Design review of the part shown in the three views and the two pictorial views. Dimensions are in mm from the part's minimum x, y and z. A direction names the side the tool comes from. Coordinates: 2 decimals unless noted, no trailing zeros. Write each loop counter-clockwise with the first axis right and the second up, starting at its lowest first coordinate (ties: lowest second). Pieces come first, ordered by that corner, then holes. Notation, with made-up numbers: (85.5, 35) - (121.5, 35) arc R23 cw to (121.5, 50) - close; hole circle Ø7 at (-13.5, -7). An arc over 180 degrees is marked (long way). Return JSON: item names as keys, results as strings. Group by question number.
(1) We need section C-C on y = 16. State the section outline as (x, z) points.
(2) We need section D-D on z = 225. State the section outline as (x, y) points, then the cut area to 3 significant figures.
(3) To check wall thickness, follow L1, parallel to X at y = 0.85, z = 125; L2, parallel to Y at x = 156.5, z = 31; L3, parallel to X at y = 2.05, z = 225. State the ranges of each line that lie inside material, in increasing order. Write a range as from..to.
(4) We need section A-A on z = 125. State the section outline as (x, y) points.
(5) We need section B-B on x = 125. State the section outline as (y, z) points, then the cut area to 3 significant figures.
(6) For pin 1 Ø1.5 at (x, z) = (125.5, 103) entering from +Y; pin 2 Ø6 at (x, z) = (123.5, 229.5) entering from -Y; pin 3 Ø1.5 at (y, z) = (19.5, 111) entering from +X, all flat-tipped, find the tip position at first contact; note any pin that passes through.
(7) Tool access review of the marked faces 1 and 2: name each direction out of +Z, -Z, +X, -X, +Y, -Y from which nothing blocks a thin tool from reaching the whole face with its end or side.
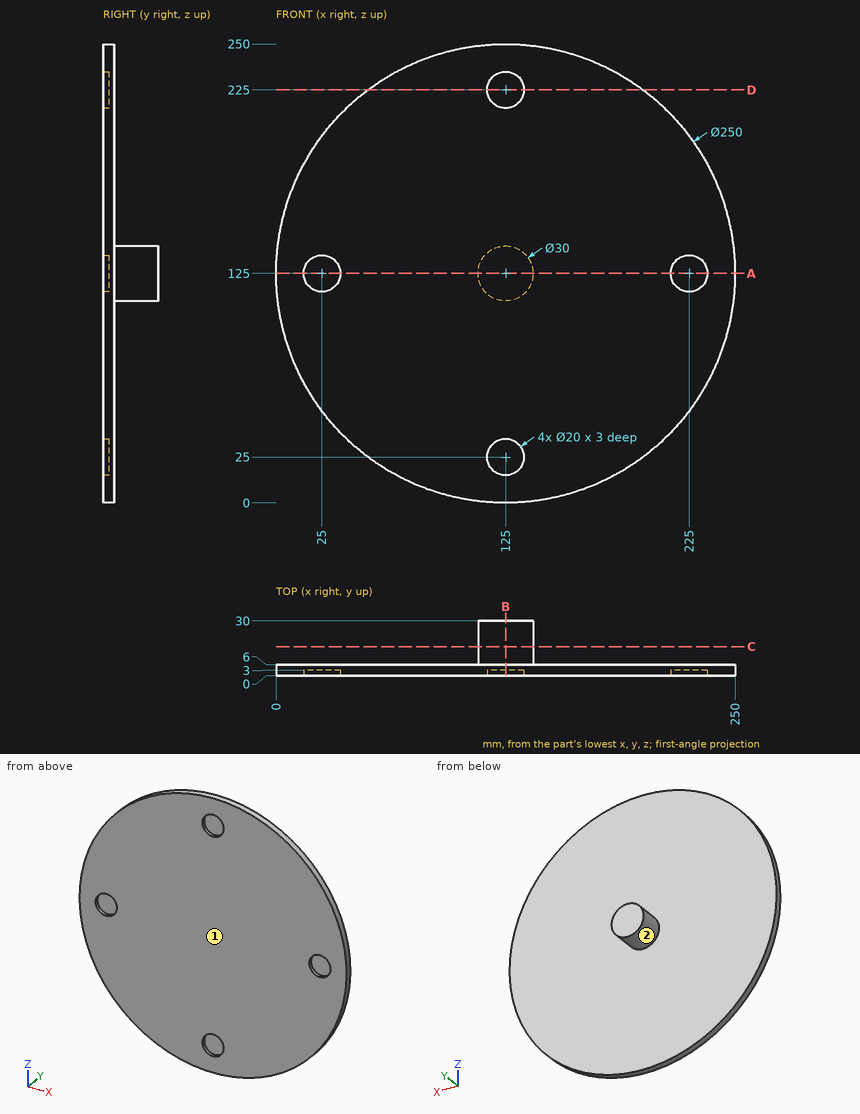
Ans:
{
 "1": {"outline": "circle Ø30 at (125, 125)"},
 "2": {"outline": "(50, 0) - (115, 0) - (115, 3) - (135, 3) - (135, 0) - (200, 0) - (200, 6) - (50, 6) - close", "area": "840 mm²"},
 "3": {"L1": "0..15, 35..215, 235..250", "L2": "0..6", "L3": "50..115, 135..200"},
 "4": {"outline": "(0, 0) - (15, 0) - (15, 3) - (35, 3) - (35, 0) - (215, 0) - (215, 3) - (235, 3) - (235, 0) - (250, 0) - (250, 6) - (140, 6) - (140, 30) - (110, 30) - (110, 6) - (0, 6) - close"},
 "5": {"outline": "(0, 0) - (6, 0) - (6, 110) - (30, 110) - (30, 140) - (6, 140) - (6, 250) - (0, 250) - (0, 235) - (3, 235) - (3, 215) - (0, 215) - (0, 35) - (3, 35) - (3, 15) - (0, 15) - close", "area": "2,100 mm²"},
 "6": {"pin 1": "y = 6", "pin 2": "y = 3", "pin 3": "x = 132.03"},
 "7": {"face 1": "+Z, -Z, +X, -X, -Y", "face 2": "+Y"}
}
